```python
from build123d import *

# Parameters (mm, degrees)
F0_W     = 36
F0_H     = 21
F0_R     = 4.1
F1_DEPTH = 5
F2_R     = 5
F4_DEPTH = 5
F5_R     = 1.25
F6_DEPTH = 5


# Not quite as in the source:
# - a pattern or mirror of a feature is missing from the dataset's text; its kind, count and spacing are read off the source's solid


with BuildPart() as f1:
    # F0 (on Top) → F1 (new body)
    with BuildSketch(Plane.XY):
        with BuildLine():
            Line((-21, 13.5), (-21, 10.5))
            Line((-21, 10.5), (-21, -13.5))
            Line((-21, -13.5), (21, -13.5))
            Line((21, -13.5), (21, 10.5))
            Line((21, 10.5), (21.0088081658, 13.5))
            Line((21.0088081658, 13.5), (7.0901421979, 13.5))
            Line((7.0901421979, 13.5), (7.0901421979, 20.8740101776))
            ThreePointArc((7.0901421979, 20.8740101776), (0, 27.6), (-7.0901421979, 20.8740101776))
            Line((-7.0901421979, 20.8740101776), (-7.0901421979, 13.5))
            Line((-7.0901421979, 13.5), (-21, 13.5))
        make_face()
        Rectangle(F0_W, F0_H, mode=Mode.SUBTRACT)
        with Locations((0, 20.5)):
            Circle(F0_R, mode=Mode.SUBTRACT)
    extrude(amount=F1_DEPTH)

    # F2
    f2_edges = [f1.edges().sort_by_distance(p)[0] for p in [
        (-7.090142, 13.5, 2.5),
        (7.090142, 13.5, 2.5),
        (21.008808, 13.5, 2.5),
        (-21, 13.5, 2.5),
        (-21, -13.5, 2.5),
        (21, -13.5, 2.5),
    ]]
    fillet(f2_edges, radius=F2_R)

    # F3 (on face) → F4 (join, through all)
    with BuildSketch(Plane.XY.offset(5)):
        with BuildLine():
            ThreePointArc((-16.9974730705, -13.3994946141), (-15.0502685736, -15.4993681678), (-13, -13.5))
            Line((-13, -13.5), (-16, -13.5))
            ThreePointArc((-16, -13.5), (-16.5012618724, -13.4748102009), (-16.9974730705, -13.3994946141))
        make_face()
    f4 = extrude(amount=-F4_DEPTH)

    # F4_copies: F4 across plane
    add(f4.mirror(Plane(origin=(0, 0, 0), x_dir=(0, 0, 1), z_dir=(1, 0, 0))))

    # F5 (on face) → F6 (cut, through all)
    with BuildSketch(Plane.XY.offset(5)):
        with Locations((-15, -13.5)):
            Circle(F5_R)
    f6 = extrude(amount=-F6_DEPTH, mode=Mode.SUBTRACT)

    # F6_copies: F6 across plane
    add(f6.mirror(Plane(origin=(0, 0, 0), x_dir=(0, 0, 1), z_dir=(1, 0, 0))), mode=Mode.SUBTRACT)


solid = f1.part
```
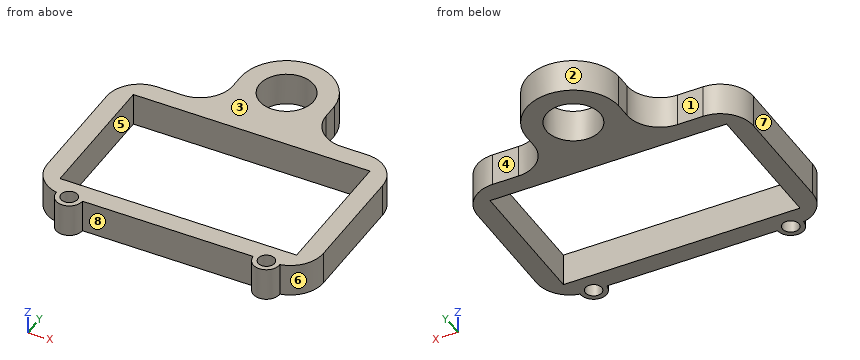
Work out the finished part from the listing and answer in its coordinate system (mm). Face numbers are marked on the shaded views. A direction names the side the tool comes from. Coordinates: 2 decimals unless noted, no trailing zeros. Write each loop counter-clockwise with the first axis right and the second up, starting at its lowest first coordinate (ties: lowest second). Pieces come first, ordered by that corner, then holes.
Q1. Which of the six approach directions +Z, -Z, +X, -X, +Y, -Y give full straight-line access (tool end or side, diameter ignored) to the marked faces 1, 2, 3, 4 and 5?
Q2. Find the intervals of material crossed by line 1 (Y direction, x = -15, z = 3); line 2 (X direction, y = -1, z = 2.85); line 3 (Y direction, x = 1.5, z = 3.9), in increasing order.
Q3. Determine the mould class of the marked faces 6, 7 and 8 for opening direction X: released by +X, released by -X, zero draft, split by the parting line, or undercut.
Q4. A cutting plane is placed at D-D, the plane z = 0.7. State how many separate pieces and enclosed holes the cut face has, then the cut area to 3 significant figures.
Q5. A cutting plane is placed at B-B, the plane x = -10. Give the vertices of the cut face in (y, z), then the cut area to 3 significant figures.
Q6. Each of these flat-tipped pins is pushed along its axis until it touches: pin 1 Ø1.2 at (y, z) = (19, 1.5) entering from -X; pin 2 Ø1.5 at (x, y) = (-15, -13.5) entering from +Z; pin 3 Ø0.7 at (y, z) = (19.5, 2.5) entering from +X. Where does it stop, or does it pass through?
Q7. A cutting plane is placed at C-C, the plane x = -15. Give the vertices of the cut face in (y, z), then the cut area to 3 significant figures.
Q8. A cutting plane is placed at A-A, the plane y = 4. Give the vertices of the cut face in (x, z).
Findings below:
1. face 1: +Z, -Z, -X, +Y
1. face 2: +Z, -Z, +Y
1. face 3: +Z, +X, -X, +Y, -Y
1. face 4: +Z, -Z, +X, +Y
1. face 5: +Z, -Z
2. line 1: y = -15.5 to -14.75, -12.25 to -10.5, 10.5 to 13.5
2. line 2: x = -21 to -18, 18 to 21
2. line 3: y = -13.5 to -10.5, 10.5 to 16.68, 24.32 to 27.44
3. face 6: released by +X
3. face 7: released by -X
3. face 8: undercut
4. separate pieces: 1
4. enclosed holes: 4
4. area: 496 mm2
5. outline: (-13.5, 0) - (-10.5, 0) - (-10.5, 5) - (-13.5, 5) - close; (10.5, 0) - (13.96, 0) - (13.96, 5) - (10.5, 5) - close
5. area: 32.3 mm2
6. pin 1: stops at x = -7.09
6. pin 2: passes through
6. pin 3: stops at x = 7.09
7. outline: (-15.5, 0) - (-14.75, 0) - (-14.75, 5) - (-15.5, 5) - close; (-12.25, 0) - (-10.5, 0) - (-10.5, 5) - (-12.25, 5) - close; (10.5, 0) - (13.5, 0) - (13.5, 5) - (10.5, 5) - close
7. area: 27.5 mm2
8. outline: (-21, 0) - (-18, 0) - (-18, 5) - (-21, 5) - close; (18, 0) - (21, 0) - (21, 5) - (18, 5) - close
